from build123d import *

# Parameters (mm, degrees)
BOX002_W          = 33
BOX002_H          = 33
BOX002_DEPTH      = 58
CYLINDER005_R     = 7.5
CYLINDER005_DEPTH = 10


with BuildPart() as cube002:
    # Box002 → Box002 (new body)
    with BuildSketch(Plane(origin=(-16.5, -16.5, 3), x_dir=(1, 0, 0), z_dir=(0, 0, 1))):
        with Locations((16.5, 16.5)):
            Rectangle(BOX002_W, BOX002_H)
    extrude(amount=BOX002_DEPTH)


with BuildPart() as laser_module:
    # Cylinder005 → Cylinder005 (new body)
    with BuildSketch(Plane.XY.offset(-2)):
        Circle(CYLINDER005_R)
    extrude(amount=CYLINDER005_DEPTH)

    # Fusion006: union Cube002
    add(cube002.part)


with BuildPart() as laser_module_1:
    # Fusion006 placement: moved
    add(laser_module.part.moved(Location((0, 0, -2))))


solid = laser_module_1.part
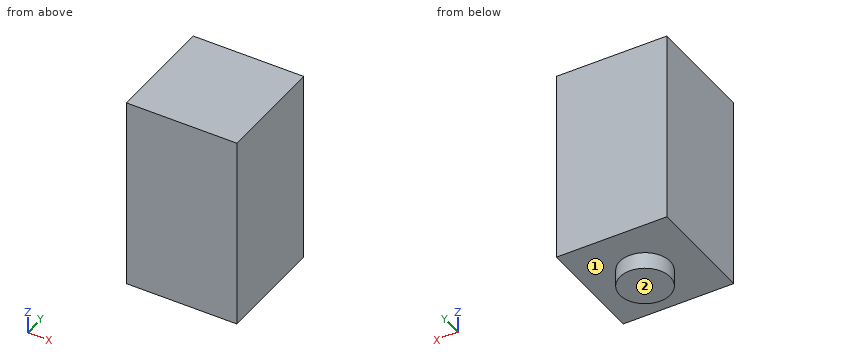
Work out the finished part from the listing and answer in its coordinate system (mm). Face numbers are marked on the shaded views. A direction names the side the tool comes from. Give positions to 0.01 mm unless a question says otherwise; leave off trailing zeros. Order: outer loops, then holes, each group sorted by start corner. A loop starts at its lowest first (then second) coordinate and runs counter-clockwise, first axis right, second up. Notation, with made-up numbers: (-23, 59) -> (-19, 59) arc R8 ccw to (-19, 70) -> close; hole circle Ø8 at (-31.5, -7). An arc over 180 degrees is marked (long way). Answer as a JSON object with one key per item and string values. Group by question number.
1. Consider line 1 along Z through (x, y) = (9, 11.5). Determine where the line is inside the solid, lowest interval first. Write a range as [from, to].
2. Section B-B on x = -6 is taken. Determine the outline of the cut face in (y, z).
3. Section A-A on y = 0 is taken. Determine the outline of the cut face in (x, z).
4. Section C-C on x = 11.5 is taken. Determine the outline of the cut face in (y, z).
5. A tool of negligible diameter and unlimited length cuts with its end or side. For the marked faces 1 and 2, from which of +Z, -Z, +X, -X, +Y, -Y can it reach the whole face along a straight path? Write none if from no direction.
6. A flat-ended cylindrical pin translates along its axis: pin 1 Ø3 at (x, y) = (-10.5, 3) entering from -Z. Find the tip coordinate at first contact, or state that the pin passes through.
Result sheet:
{
 "1": {"line 1": "z = [1, 59]"},
 "2": {"outline": "(-16.5, 1) -> (-4.5, 1) -> (-4.5, -4) -> (4.5, -4) -> (4.5, 1) -> (16.5, 1) -> (16.5, 59) -> (-16.5, 59) -> close"},
 "3": {"outline": "(-16.5, 1) -> (-7.5, 1) -> (-7.5, -4) -> (7.5, -4) -> (7.5, 1) -> (16.5, 1) -> (16.5, 59) -> (-16.5, 59) -> close"},
 "4": {"outline": "(-16.5, 1) -> (16.5, 1) -> (16.5, 59) -> (-16.5, 59) -> close"},
 "5": {"face 1": "-Z", "face 2": "-Z, +X, -X, +Y, -Y"},
 "6": {"pin 1": "stops at z = 1"}
}
